```python
from build123d import *

# Parameters (mm, degrees)
P_IDAT_VYSUNUT_M1_DEPTH                     = 53
ODEBRAT_VYSUNUT_M1_DEPTH                    = 35
V_LCOV_START                                = 38.6
V_LCOV_ZAHLOUBEN_PRO_M6_ROUBY_S_V_2_R       = 5.5
V_LCOV_ZAHLOUBEN_PRO_M6_ROUBY_S_VNIT_DEPTH  = 25.392214676
V_LCOV_ZAHLOUBEN_PRO_M6_ROUBY_S_V_3_O_R     = 3.3
V_LCOV_ZAHLOUBEN_PRO_M6_ROUBY_S_V_3_DEPTH   = 38.6
V_LCOV_START_2                              = 13.6
V_LCOV_ZAHLOUBEN_PRO_M6_ROUBY_S_V_4_O_R     = 5.5
V_LCOV_ZAHLOUBEN_PRO_M6_ROUBY_S_V_4_DEPTH   = 18.891616585
V_LCOV_ZAHLOUBEN_PRO_M6_ROUBY_S_V_5_R       = 3.3
V_LCOV_ZAHLOUBEN_PRO_M6_ROUBY_S_V_4_2_DEPTH = 13.6
M8_Z_VIT1_D                                 = 6.8
M8_Z_VIT1_DEPTH                             = 15
M8_Z_VIT1_CSINK_D                           = 8.05
M8_Z_VIT1_CSINK_ANGLE                       = 90
M8_Z_VIT1_TIP                               = 2.042926105


# Read off the part's stored shape, not the designer's step: Válcové zahloubení pro M6 šrouby s vnitřním šestihranem1, Válcové zahloubení pro M6 šrouby s vnitřním šestihranem2
with BuildPart() as part:
    # Skica1 → Přidat vysunutím1 (new, symmetric)
    with BuildSketch(Plane.XY):
        Polygon((61.822124963, 0), (25.791252921, 60), (-25.791252921, 60), (-61.822124963, 0), align=None)
        Polygon((-25.791252921, 60), (25.791252921, 60), (61.822124963, 0), (81.822124963, 0), (81.822124963, 20), (35.791252921, 70), (-35.791252921, 70), (-81.822124963, 20), (-81.822124963, 0), (-61.822124963, 0), align=None)
    extrude(amount=P_IDAT_VYSUNUT_M1_DEPTH, both=True)

    # Skica1<3> → Odebrat vysunutím1 (cut, symmetric)
    with BuildSketch(Plane.XY):
        Polygon((61.822124963, 0), (25.791252921, 60), (-25.791252921, 60), (-61.822124963, 0), align=None)
    extrude(amount=ODEBRAT_VYSUNUT_M1_DEPTH, both=True, mode=Mode.SUBTRACT)

    # V_lcov_ zahlouben_ pro M6 _rouby s v 2 → V_lcov_ zahlouben_ pro M6 _rouby s vnit (cut)
    with BuildSketch(Plane(origin=(0, 0, 0), x_dir=(1, 0, 0), z_dir=(0, 1, 0)).offset(V_LCOV_START)):
        with Locations((46.822124963, 47)):
            Circle(V_LCOV_ZAHLOUBEN_PRO_M6_ROUBY_S_V_2_R)
        with Locations((-46.822124963, -47)):
            Circle(V_LCOV_ZAHLOUBEN_PRO_M6_ROUBY_S_V_2_R)
        with Locations((46.822124963, -47)):
            Circle(V_LCOV_ZAHLOUBEN_PRO_M6_ROUBY_S_V_2_R)
        with Locations((-46.822124963, 47)):
            Circle(V_LCOV_ZAHLOUBEN_PRO_M6_ROUBY_S_V_2_R)
    extrude(amount=V_LCOV_ZAHLOUBEN_PRO_M6_ROUBY_S_VNIT_DEPTH, mode=Mode.SUBTRACT)

    # V_lcov_ zahlouben_ pro M6 _rouby s v 3 o → V_lcov_ zahlouben_ pro M6 _rouby s v 3 (cut)
    with BuildSketch(Plane(origin=(0, 0, 0), x_dir=(1, 0, 0), z_dir=(0, 1, 0))):
        with Locations((46.822124963, 47)):
            Circle(V_LCOV_ZAHLOUBEN_PRO_M6_ROUBY_S_V_3_O_R)
        with Locations((-46.822124963, -47)):
            Circle(V_LCOV_ZAHLOUBEN_PRO_M6_ROUBY_S_V_3_O_R)
        with Locations((46.822124963, -47)):
            Circle(V_LCOV_ZAHLOUBEN_PRO_M6_ROUBY_S_V_3_O_R)
        with Locations((-46.822124963, 47)):
            Circle(V_LCOV_ZAHLOUBEN_PRO_M6_ROUBY_S_V_3_O_R)
    extrude(amount=V_LCOV_ZAHLOUBEN_PRO_M6_ROUBY_S_V_3_DEPTH, mode=Mode.SUBTRACT)

    # V_lcov_ zahlouben_ pro M6 _rouby s v 4 o → V_lcov_ zahlouben_ pro M6 _rouby s v 4 (cut)
    with BuildSketch(Plane(origin=(0, 0, 0), x_dir=(1, 0, 0), z_dir=(0, 1, 0)).offset(V_LCOV_START_2)):
        with Locations((75.822124963, 25)):
            Circle(V_LCOV_ZAHLOUBEN_PRO_M6_ROUBY_S_V_4_O_R)
        with Locations((-75.822124963, -25)):
            Circle(V_LCOV_ZAHLOUBEN_PRO_M6_ROUBY_S_V_4_O_R)
        with Locations((75.822124963, -25)):
            Circle(V_LCOV_ZAHLOUBEN_PRO_M6_ROUBY_S_V_4_O_R)
        with Locations((-75.822124963, 25)):
            Circle(V_LCOV_ZAHLOUBEN_PRO_M6_ROUBY_S_V_4_O_R)
    extrude(amount=V_LCOV_ZAHLOUBEN_PRO_M6_ROUBY_S_V_4_DEPTH, mode=Mode.SUBTRACT)

    # V_lcov_ zahlouben_ pro M6 _rouby s v 5 → V_lcov_ zahlouben_ pro M6 _rouby s v 4 2 (cut)
    with BuildSketch(Plane(origin=(0, 0, 0), x_dir=(1, 0, 0), z_dir=(0, 1, 0))):
        with Locations((75.822124963, 25)):
            Circle(V_LCOV_ZAHLOUBEN_PRO_M6_ROUBY_S_V_5_R)
        with Locations((-75.822124963, -25)):
            Circle(V_LCOV_ZAHLOUBEN_PRO_M6_ROUBY_S_V_5_R)
        with Locations((75.822124963, -25)):
            Circle(V_LCOV_ZAHLOUBEN_PRO_M6_ROUBY_S_V_5_R)
        with Locations((-75.822124963, 25)):
            Circle(V_LCOV_ZAHLOUBEN_PRO_M6_ROUBY_S_V_5_R)
    extrude(amount=V_LCOV_ZAHLOUBEN_PRO_M6_ROUBY_S_V_4_2_DEPTH, mode=Mode.SUBTRACT)

    # M8 závit1
    with Locations(Plane(origin=(0, 70, 0), x_dir=(1, 0, 0), z_dir=(0, 1, 0))):
        with Locations((-23.791252921, 33)):
            CounterSinkHole(M8_Z_VIT1_D / 2, M8_Z_VIT1_CSINK_D / 2, depth=M8_Z_VIT1_DEPTH, counter_sink_angle=M8_Z_VIT1_CSINK_ANGLE)
            with Locations((0, 0, -(M8_Z_VIT1_DEPTH + M8_Z_VIT1_TIP / 2))):  # 118° drill point
                Cone(0, M8_Z_VIT1_D / 2, M8_Z_VIT1_TIP, mode=Mode.SUBTRACT)

    # Skica12 → Odebrat rotací1 (revolve, cut)
    with BuildSketch(Plane.XZ):
        Polygon((0, 61), (29, 61), (29, 51), (31, 51), (31, -51), (29, -51), (29, -61), (0, -61), align=None)
    revolve(axis=Axis((0, 0, -71.132425853), (0, 0, 1)), mode=Mode.SUBTRACT)


solid = part.part
```
Here's how the part is built. I have some questions about the finished solid (model axes, mm). A direction names the side the tool comes from. Coordinates: 2 decimals unless noted, no trailing zeros. Write each loop counter-clockwise with the first axis right and the second up, starting at its lowest first coordinate (ties: lowest second). Pieces come first, ordered by that corner, then holes. Notation, with made-up numbers: (-15, -20.75) - (23, -20.75) arc R6 cw to (23, -9.75) - close; hole circle Ø11 at (-25.75, 61). An arc over 180 degrees is marked (long way). One line per item, written item: value.
1) Suppose I cut it at A-A on z = -25. Write out the boundary of the cut face in (x, y).
Model answer:
outline: (-81.82, 0) - (-79.12, 0) - (-79.12, 13.6) - (-81.32, 13.6) - (-81.32, 20.54) - (-81.82, 20) - close; (-72.52, 0) - (-61.82, 0) - (-25.79, 60) - (25.79, 60) - (61.82, 0) - (72.52, 0) - (72.52, 13.6) - (70.32, 13.6) - (70.32, 32.49) - (35.79, 70) - (-35.79, 70) - (-70.32, 32.49) - (-70.32, 13.6) - (-72.52, 13.6) - close; (79.12, 0) - (81.82, 0) - (81.82, 20) - (81.32, 20.54) - (81.32, 13.6) - (79.12, 13.6) - close
2) I need wall thicknesses on line 1 along Z through (x, y) = (18, 46.5); line 2 along X through (y, z) = (13.5, -47); line 3 along X through (y, z) = (53.75, -47). Which ranges of each line are inside material? Lowest first, please.
Model answer:
line 1: z = -53 to -35, 35 to 53
line 2: x = -81.82 to -50.12, -43.52 to -27.91, 27.91 to 43.52, 50.12 to 81.82
line 3: x = -41.32 to 41.32
3) Suppose I cut it at C-C on z = 9.5. Write out the boundary of the cut face in (x, y).
Model answer:
outline: (-81.82, 0) - (-61.82, 0) - (-25.79, 60) - (25.79, 60) - (61.82, 0) - (81.82, 0) - (81.82, 20) - (35.79, 70) - (-35.79, 70) - (-81.82, 20) - close
4) On a 3-axis mill with a long thin cutter (end or side, diameter ignored), from which of +Z, -Z, +X, -X, +Y, -Y can I reach the whole of each face in a straight line? I mean faces 1 (the cylindrical face through (-70.742, 20.814, -22.893)), 2 (the cylindrical face through (0.682, 30.993, 42.888)), 3 (the flat face through (-81.822, 10, 1)). Say none if no direction works.
Model answer:
face 1: +Y
face 2: -Y
face 3: +Z, -Z, -X, +Y, -Y
5) We'd pull the mould along Z, two halves only. Please class faces 4 (the flat face through (79.4, 13.6, 24.9)), 5 (the cylindrical face through (0.638, 28.993, -52.014)): pulls with the +Z half, pulls with the -Z half, needs draft (parallel to the pull), parting line crosses it, or undercut.
Model answer:
face 4: undercut
face 5: needs draft
6) Suppose I cut it at B-B on y = 6. State how many separate pieces and enclosed holes the cut face has, and give its area (3 significant figures).
Model answer:
separate pieces: 2
enclosed holes: 8
area: 6,750 mm²
7) I'm going to push flat-ended pins straight in: P1, Ø14.5, axis at x = -46.82, z = 47, coming from the +Y side; P2, Ø9, axis at x = 48, z = -49, coming from the +Y side; P3, Ø9, axis at x = -75, z = 25.5, coming from the +Y side; P4, Ø5.5, axis at x = -75.82, z = -25, coming from the +Y side. Where does each tip first touch, or does it pass through?
Model answer:
P1: stops at y = 65.9
P2: stops at y = 60.3
P3: stops at y = 13.6
P4: passes through
